For this review, take the finished solid that the model builds, in its own axes (mm). A direction names the side the tool comes from. Coordinates: 2 decimals unless noted, no trailing zeros. Loops run counter-clockwise (first coordinate to the right, second up) from the corner with the lowest first, then second, coordinate; pieces in that order, holes last. Notation, with made-up numbers: (-5.75, 50) - (3.25, 50) arc R21 ccw to (3.25, 55) - close; hole circle Ø7 at (27, -19). An arc over 180 degrees is marked (long way). One line per item, written item: value. Start each with the question number.
1. Insertion check: pin 1 (8 mm diameter, centred on x = 17.5, z = -42.5, fed in from +Y); pin 2 (1 mm diameter, centred on x = 14, y = 2, fed in from -Z); pin 3 (1.5 mm diameter, centred on x = 6.5, y = 6.5, fed in from -Z); pin 4 (6 mm diameter, centred on x = -10, y = 7, fed in from +Z). Each pin has a flat end and moves straight along its axis. Give the tip position at first contact, or say it passes through.
2. Take a section at B-B, the plane z = -57.5. State the section outline as (x, y) points.
3. Take a section at C-C, the plane y = -11.25. State the section outline as (x, z) points.
4. Take a section at A-A, the plane x = 17.5. State the section outline as (y, z) points, and give its area (3 significant figures).
5. For faces 1 (the face through (0, 0, -95)), 2 (the face through (19, 0, -50)), 3 (the face through (-18, 0, -50)), 4 (the face through (-7.493, -0.33, -17.255)), 5 (the face through (7.154, -2.253, -82.255)), list the 3-axis set-ups (+Z, -Z, +X, -X, +Y, -Y) from which the entire face can be reached by the end or side of a thin tool; tool diameter is ignored.
6. The part is to be moulded in two halves that separate along X. For faces 6 (the face through (10.556, 0.46, -50.21)), 7 (the face through (0, -15, -50)), 8 (the face through (-25, -7, -50)), 9 (the face through (-18.46, -7.4, -55.19)), say which applies: released by +X, released by -X, zero draft, split by the parting line, or undercut.
7. Take a section at D-D, the plane x = 0. State the section outline as (y, z) points.
8. To check wall thickness, follow line 1 (X direction, y = -5.5, z = -57.5); line 2 (Y direction, x = -14.5, z = -40.5); line 3 (Z direction, x = 20.5, y = -9). State the ranges of each line that lie inside material, in increasing order. Write a range as from..to.
```python
from build123d import *

# Parameters (mm, degrees)
BOSS_EXTRUDE1_DEPTH      = 15
BOSS_EXTRUDE1_DEPTH_BACK = 15
SKETCH6_R                = 2.5
CUT_EXTRUDE2_DEPTH       = 25
CUT_EXTRUDE3_DEPTH       = 35
CUT_EXTRUDE3_DEPTH_BACK  = 30
SKETCH8_R                = 2.5


with BuildPart() as part:
    # Sketch1 → Revolve1 (revolve)
    with BuildSketch(Plane(origin=(0, 0, 0), x_dir=(1, 0, 0), z_dir=(0, 1, 0))):
        Polygon((0, 90), (0, 100), (2, 100), (7.5, 100), (7.5, 65), (9, 65), (9, 35), (7.5, 35), (7.5, 0), (0, 0), align=None)
    revolve(axis=Axis((0, 0, -90), (0, 0, -1)))

    # Sketch5 → Boss-Extrude1 (add, two sides: drawn at the far end of the back side and taken through both)
    with BuildSketch(Plane.XY.offset(-50).offset(-BOSS_EXTRUDE1_DEPTH_BACK)):
        with BuildLine():
            Line((-25, -10), (-25, -15))
            Line((-25, -15), (25, -15))
            Line((25, -15), (25, -10))
            Line((25, -10), (25, 0))
            Line((25, 0), (20, 0))
            Line((20, 0), (12.5, 0))
            Line((12.5, 0), (11.832159566, 0))
            ThreePointArc((11.832159566, 0), (10.541165117, 0.472474768), (9.860132972, 1.666666667))
            ThreePointArc((9.860132972, 1.666666667), (0, 10), (-9.860132972, 1.666666667))
            ThreePointArc((-9.860132972, 1.666666667), (-10.541165117, 0.472474768), (-11.832159566, 0))
            Line((-11.832159566, 0), (-12.5, 0))
            Line((-12.5, 0), (-20, 0))
            Line((-20, 0), (-25, 0))
            Line((-25, 0), (-25, -10))
        make_face()
    extrude(amount=BOSS_EXTRUDE1_DEPTH + BOSS_EXTRUDE1_DEPTH_BACK)

    # Sketch6 → Cut-Extrude2 (cut)
    with BuildSketch(Plane(origin=(0, 0, 0), x_dir=(1, 0, 0), z_dir=(0, 1, 0))):
        with Locations(Location((-17.5, 57.5, 0), (0, 0, 270))):
            Circle(SKETCH6_R)
        with Locations(Location((17.5, 57.5, 0), (0, 0, 270))):
            Circle(SKETCH6_R)
        with Locations(Location((17.5, 42.5, 0), (0, 0, 270))):
            Circle(SKETCH6_R)
        with Locations(Location((-17.5, 42.5, 0), (0, 0, 270))):
            Circle(SKETCH6_R)
    extrude(amount=-CUT_EXTRUDE2_DEPTH, mode=Mode.SUBTRACT)

    # Sketch8 → Cut-Extrude3 (cut, two sides: drawn at the far end of the back side and taken through both)
    with BuildSketch(Plane(origin=(0, 0, 0), x_dir=(1, 0, 0), z_dir=(0, 1, 0)).offset(-CUT_EXTRUDE3_DEPTH_BACK)):
        with Locations(Location((0, 92.5, 0), (0, 0, 270))):
            Circle(SKETCH8_R)
    extrude(amount=CUT_EXTRUDE3_DEPTH + CUT_EXTRUDE3_DEPTH_BACK, mode=Mode.SUBTRACT)


solid = part.part
```
Solutions:
1. pin 1: y = 0
1. pin 2: through
1. pin 3: z = -65
1. pin 4: z = -35
2. outline: (-25, -15) - (-20, -15) - (-20, 0) - (-25, 0) - close; (-15, -15) - (15, -15) - (15, 0) - (11.83, 0) arc R2 cw to (9.86, 1.67) arc R10 ccw to (-9.86, 1.67) arc R2 cw to (-11.83, 0) - (-15, 0) - close; (20, -15) - (25, -15) - (25, 0) - (20, 0) - close
3. outline: (-25, -65) - (25, -65) - (25, -35) - (-25, -35) - close; hole circle Ø5 at (-17.5, -57.5); hole circle Ø5 at (-17.5, -42.5); hole circle Ø5 at (17.5, -57.5); hole circle Ø5 at (17.5, -42.5)
4. outline: (-15, -65) - (0, -65) - (0, -60) - (-15, -60) - close; (-15, -55) - (0, -55) - (0, -45) - (-15, -45) - close; (-15, -40) - (0, -40) - (0, -35) - (-15, -35) - close
4. area: 300 mm2
5. face 1: +Y, -Y
5. face 2: +Z, -Z, +X, +Y
5. face 3: +Z, -Z, -X, +Y
5. face 4: +Z
5. face 5: -Z
6. face 6: released by +X
6. face 7: zero draft
6. face 8: released by -X
6. face 9: undercut
7. outline: (-15, -65) - (-7.5, -65) - (-7.5, -90) - (7.5, -90) - (7.5, -65) - (10, -65) - (10, -35) - (7.5, -35) - (7.5, 0) - (-7.5, 0) - (-7.5, -35) - (-15, -35) - close; (-7.5, -100) - (7.5, -100) - (7.5, -95) - (-7.5, -95) - close
8. line 1: -25..-20, -15..15, 20..25
8. line 2: -15..0
8. line 3: -65..-35
